Input: part model. Units: mm. Frame: model coordinates. Coordinates: 2 decimals unless noted, no trailing zeros. Order: outer loops, then holes, each group sorted by start corner. A loop starts at its lowest first (then second) coordinate and runs counter-clockwise, first axis right, second up. Notation, with made-up numbers: (35, 52) - (74, 52) arc R25 cw to (74, 80) - close; hole circle Ø6 at (-26, 74). An arc over 180 degrees is marked (long way). One line per question, with ' | ' between items.
from build123d import *

# Parameters (mm, degrees)
SKETCH1_W      = 203.2
SKETCH1_H      = 203.2
EXTRUDE1_DEPTH = 6.35
SKETCH2_R      = 6.1468
EXTRUDE2_DEPTH = 144.824345992
SKETCH3_R      = 1.4097
EXTRUDE3_DEPTH = 144.824345992
SKETCH4_W      = 0.79375
SKETCH4_H      = 6.35
EXTRUDE4_DEPTH = 6.35
SKETCH5_R      = 2.8575
EXTRUDE5_DEPTH = 144.824345992


with BuildPart() as part:
    # Sketch1 → Extrude1 (new body)
    with BuildSketch(Plane.XY):
        Rectangle(SKETCH1_W, SKETCH1_H)
    extrude(amount=EXTRUDE1_DEPTH)

    # Sketch2 → Extrude2 (cut, through all)
    with BuildSketch(Plane.XY.offset(6.35)):
        Circle(SKETCH2_R)
    extrude(amount=-EXTRUDE2_DEPTH, mode=Mode.SUBTRACT)

    # Sketch3 → Extrude3 (cut, through all)
    with BuildSketch(Plane.XY.offset(6.35)):
        with Locations((-47.625, -82.48891971)):
            Circle(SKETCH3_R)
        with Locations((47.625, -82.48891971)):
            Circle(SKETCH3_R)
    extrude(amount=-EXTRUDE3_DEPTH, mode=Mode.SUBTRACT)

    # Sketch4 → Extrude4 (cut)
    with BuildSketch(Plane.XY.offset(6.35)):
        with Locations((0, -98.425)):
            Rectangle(SKETCH4_W, SKETCH4_H)
    extrude(amount=-EXTRUDE4_DEPTH, mode=Mode.SUBTRACT)

    # Sketch5 → Extrude5 (cut, through all)
    with BuildSketch(Plane.XY.offset(6.35)):
        with Locations((-79.82293888, 72.673935689)):
            Circle(SKETCH5_R)
        with Locations((72.673935689, 79.82293888)):
            Circle(SKETCH5_R)
        with Locations((-72.673935689, -79.82293888)):
            Circle(SKETCH5_R)
        with Locations((79.82293888, -72.673935689)):
            Circle(SKETCH5_R)
    extrude(amount=-EXTRUDE5_DEPTH, mode=Mode.SUBTRACT)


solid = part.part
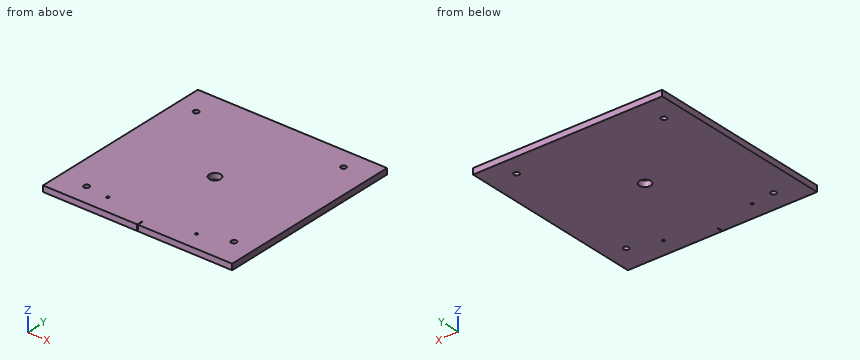
Item 1: Section B-B on x = -3.5. Return the cut outline in (y, z), and give its area (3 significant figures).
Data:
outline: (-101.6, 0) - (-5.05, 0) - (-5.05, 6.35) - (-101.6, 6.35) - close; (5.05, 0) - (101.6, 0) - (101.6, 6.35) - (5.05, 6.35) - close | area: 1,230 mm^2
Item 2: Section A-A on y = 0. Return the cut outline in (x, z).
Data:
outline: (-101.6, 0) - (-6.15, 0) - (-6.15, 6.35) - (-101.6, 6.35) - close; (6.15, 0) - (101.6, 0) - (101.6, 6.35) - (6.15, 6.35) - close
Item 3: Ray query, line 1 (X direction, y = 72.5, z = 3.75); line 2 (Y direction, x = 0.5, z = 1); line 3 (X direction, y = -72, z = 6). Return the intervals inside material, ascending.
Data:
line 1: -101.6 to -82.68, -76.97 to 101.6 | line 2: -101.6 to -6.13, 6.13 to 101.6 | line 3: -101.6 to 77.05, 82.6 to 101.6
